from build123d import *

# Parameters (mm, degrees)
SKETCH1_W           = 12
SKETCH1_H           = 17
BOSS_EXTRUDE1_DEPTH = 3
SKETCH3_W           = 1
SKETCH3_H           = 11
CUT_EXTRUDE1_DEPTH  = 16
CUT_EXTRUDE2_REACH  = 23.024
SKETCH2_W           = 5
SKETCH2_H           = 9


with BuildPart() as part:
    # Sketch1 → Boss-Extrude1 (new body)
    with BuildSketch(Plane(origin=(0, 0, 0), x_dir=(0, 0, -1), z_dir=(1, 0, 0))):
        with Locations((6, -8.5)):
            Rectangle(SKETCH1_W, SKETCH1_H)
    extrude(amount=BOSS_EXTRUDE1_DEPTH)

    # Sketch3 → Cut-Extrude1 (cut)
    with BuildSketch(Plane(origin=(0, 0, 0), x_dir=(1, 0, 0), z_dir=(0, 1, 0))):
        with Locations((1.5, 5.5)):
            Rectangle(SKETCH3_W, SKETCH3_H)
    extrude(amount=-CUT_EXTRUDE1_DEPTH, mode=Mode.SUBTRACT)

    # Sketch2 → Cut-Extrude2 (cut, up to next)
    with BuildSketch(Plane(origin=(3, 0, 0), x_dir=(0, 0, -1), z_dir=(1, 0, 0)), mode=Mode.PRIVATE) as cut_extrude2_sk1:
        with Locations((2.5, -4.5)):
            Rectangle(SKETCH2_W, SKETCH2_H)
    cut_extrude2_tool1 = extrude(cut_extrude2_sk1.sketch, amount=-CUT_EXTRUDE2_REACH, mode=Mode.PRIVATE) & part.part
    add(cut_extrude2_tool1.solids().sort_by_distance((3, -4.5, -2.5))[0], mode=Mode.SUBTRACT)


solid = part.part
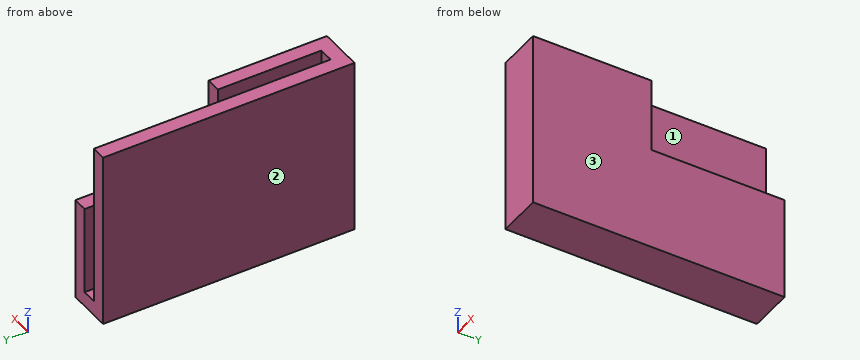
Could you check a few things on this model? Use its own coordinates, in mm. Face numbers are marked on the shaded views. Give positions to 0.01 mm unless a question says otherwise; leave off trailing zeros. Order: outer loops, then holes, each group sorted by start corner. A loop starts at its lowest first (then second) coordinate and runs counter-clockwise, first axis right, second up. Notation, with made-up numbers: (2, 15.25) - (49, 15.25) arc R20 ccw to (49, 46.25) - close; hole circle Ø3 at (50, -27). An arc over 180 degrees is marked (long way). One line per item, written item: value. Start each with the question number.
1. Imagine slicing it at B-B on y = -2.75. List the corners of the cut face in (x, z) for me, plus the area to 3 significant figures.
2. If I drill on probe 1 along X at (y, z) = (-12.5, -10.5); probe 2 along Z at (x, y) = (2.8, -7.25); probe 3 along Z at (x, y) = (1.6, -7.75), over which ranges is the centre line in solid material (lowest first)?
3. Imagine slicing it at A-A on z = -2.5. List the corners of the cut face in (x, y) for me, plus the area to 3 significant figures.
4. Imagine slicing it at C-C on x = 1.5. List the corners of the cut face in (y, z) for me.
5. Thinking about a two-plate mould opening in X: for the marked faces 1, 2 and 3, which applies, +X half, -X half, draft (parallel to the pull), parting line (faces both ways), or undercut?
6. For P1, Ø0.5, axis at x = 1.5, z = -5, coming from the +Y side; P2, Ø0.5, axis at x = 2.5, z = -1.5, coming from the +Y side; P3, Ø0.5, axis at x = 1.5, y = -7.5, coming from the +Z side, each with a flat end and sliding along its axis, tell me the tip position at first contact or that it passes through.
Values:
1. outline: (0, -12) - (3, -12) - (3, -5) - (2, -5) - (2, -11) - (1, -11) - (1, 0) - (0, 0) - close
1. area: 20.0 mm²
2. probe 1: 0 to 1, 2 to 3
2. probe 2: -12 to -5
2. probe 3: -12 to -11
3. outline: (0, -17) - (3, -17) - (3, -9) - (2, -9) - (2, -16) - (1, -16) - (1, 0) - (0, 0) - close
3. area: 26.0 mm²
4. outline: (-17, -12) - (0, -12) - (0, -11) - (-16, -11) - (-16, 0) - (-17, 0) - close
5. face 1: undercut
5. face 2: -X half
5. face 3: +X half
6. P1: y = -16
6. P2: y = -9
6. P3: z = -11
